Read the model definition and answer for the solid it produces. Units are mm, in the model's axes. Give positions to 0.01 mm unless a question says otherwise; leave off trailing zeros. Loops run counter-clockwise (first coordinate to the right, second up) from the corner with the lowest first, then second, coordinate; pieces in that order, holes last. Notation, with made-up numbers: (-0.75, -5) - (21.25, -5) arc R20 cw to (21.25, 18) - close; hole circle Ø7 at (-14, 37.25). An arc over 180 degrees is marked (long way). Use a Markdown table: item, result. Add a question column.
Item 1: A cutting plane is placed at A-A (z = 0.25). Determine the outline of the cut face in (x, y), plus the area to 3 significant figures.
Item 2: A cutting plane is placed at B-B (x = -12). Determine the outline of the cut face in (y, z).
Item 3: A cutting plane is placed at D-D (z = -2.5). Determine the outline of the cut face in (x, y), plus the area to 3 significant figures.
Item 4: This flat-tipped pin is pushed along its axis until it touches: P1, Ø2.5, axis at x = 2.67, z = -0.13, coming from the -Y side. Where does it stop, or does it pass through?
Item 5: A cutting plane is placed at C-C (y = 1.25). Determine the outline of the cut face in (x, z).
Item 6: Consider probe 1 along X at (y, z) = (1.6, -0.5); probe 2 along X at (y, z) = (0.7, 0.5); probe 3 along X at (y, z) = (1.65, 2). Determine where each line is inside the solid, lowest interval first. Write a range as [from, to].
Item 7: For a pull along Z with two mould halves and no side action, classify faces 1 (the face through (3.47, 1.01, -1.4)), 2 (the face through (-14, 1, 4.868)), 3 (the face through (-14, 2, -4)), 4 (the face through (-14, 1, -5.132)) as +Z half, -Z half, draft (parallel to the pull), parting line (faces both ways), or undercut.
from build123d import *

# Parameters (mm, degrees)
SKETCH1_W           = 40
SKETCH1_H           = 10
BOSS_EXTRUDE1_DEPTH = 2
SKETCH2_R           = 1.5
SKETCH2_R_2         = 3
CUT_EXTRUDE1_DEPTH  = 3


with BuildPart() as part:
    # Sketch1 → Boss-Extrude1 (new body)
    with BuildSketch(Plane(origin=(0, 0, 0), x_dir=(1, 0, 0), z_dir=(0, 1, 0))):
        with Locations((-13.333333333, 0.131578947)):
            Rectangle(SKETCH1_W, SKETCH1_H)
    extrude(amount=BOSS_EXTRUDE1_DEPTH)

    # Sketch2 → Cut-Extrude1 (cut, through all)
    with BuildSketch(Plane(origin=(0, 2, 0), x_dir=(1, 0, 0), z_dir=(0, 1, 0))):
        with Locations((-29.333333333, 0.131578947)):
            Circle(SKETCH2_R)
        with Locations((2.666666667, 0.131578947)):
            Circle(SKETCH2_R)
        with Locations((-13.333333333, 0.131578947)):
            Circle(SKETCH2_R_2)
    extrude(amount=-CUT_EXTRUDE1_DEPTH, mode=Mode.SUBTRACT)


solid = part.part
Geometry says:
| question | item | result |
|---|---|---|
| 1 | outline | (-33.33, 0) - (-30.78, 0) - (-30.78, 2) - (-33.33, 2) - close; (-27.88, 0) - (-16.31, 0) - (-16.31, 2) - (-27.88, 2) - close; (-10.36, 0) - (1.22, 0) - (1.22, 2) - (-10.36, 2) - close; (4.12, 0) - (6.67, 0) - (6.67, 2) - (4.12, 2) - close |
| 1 | area | 56.5 mm² |
| 2 | outline | (0, -5.13) - (2, -5.13) - (2, -2.82) - (0, -2.82) - close; (0, 2.56) - (2, 2.56) - (2, 4.87) - (0, 4.87) - close |
| 3 | outline | (-33.33, 0) - (-15.17, 0) - (-15.17, 2) - (-33.33, 2) - close; (-11.49, 0) - (6.67, 0) - (6.67, 2) - (-11.49, 2) - close |
| 3 | area | 72.6 mm² |
| 4 | P1 | through |
| 5 | outline | (-33.33, -5.13) - (6.67, -5.13) - (6.67, 4.87) - (-33.33, 4.87) - close; hole circle Ø3 at (-29.33, -0.13); hole circle Ø6 at (-13.33, -0.13); hole circle Ø3 at (2.67, -0.13) |
| 6 | probe 1 | [-33.33, -30.79], [-27.88, -16.31], [-10.36, 1.21], [4.12, 6.67] |
| 6 | probe 2 | [-33.33, -30.69], [-27.97, -16.27], [-10.4, 1.31], [4.03, 6.67] |
| 6 | probe 3 | [-33.33, -15.44], [-11.22, 6.67] |
| 7 | face 1 | undercut |
| 7 | face 2 | +Z half |
| 7 | face 3 | draft |
| 7 | face 4 | -Z half |
